```python
from build123d import *

# Parameters (mm, degrees)
SKETCH5_R           = 11.5
BOSS_EXTRUDE2_DEPTH = 3
BOSS_EXTRUDE1_DEPTH = 3
SKETCH3_W           = 6
SKETCH3_H           = 3
SKETCH3_W_2         = 3
SKETCH3_H_2         = 6
CUT_EXTRUDE1_DEPTH  = 3
SKETCH6_R           = 1.35
CUT_EXTRUDE3_DEPTH  = 3


with BuildPart() as part:
    # Sketch5 → Boss-Extrude2 (new body)
    with BuildSketch(Plane(origin=(0, 0, 0), x_dir=(1, 0, 0), z_dir=(0, 1, 0))):
        with Locations(Location((0, 0, 0), (0, 0, 270))):
            Circle(SKETCH5_R)
    extrude(amount=BOSS_EXTRUDE2_DEPTH)

    # Sketch1 → Boss-Extrude1 (add)
    with BuildSketch(Plane(origin=(0, 0, 0), x_dir=(1, 0, 0), z_dir=(0, 1, 0))):
        Polygon((0, 16), (-1.75, 11), (1.75, 11), align=None)
        Polygon((5.195191507, 15.133075867), (1.916513988, 10.97221373), (5.226874334, 9.835765588), align=None)
        Polygon((9.827403403, 12.62624815), (5.375343948, 9.755417851), (8.137335731, 7.605673356), align=None)
        Polygon((13.394663652, 8.75117053), (8.251671984, 7.481471076), (10.165990538, 4.551388402), align=None)
        Polygon((15.510404255, 3.927767794), (10.233803323, 4.396790824), (11.093002528, 1.003889893), align=None)
        Polygon((15.945351888, -1.321269528), (11.106943278, 0.835650063), (10.817915568, -2.652395663), align=None)
        Polygon((14.652373226, -6.427126794), (10.776473586, -2.81604635), (9.3705396, -6.021252993), align=None)
        Polygon((11.771582571, -10.836505146), (9.278205768, -6.162580444), (6.907720267, -8.737614132), align=None)
        Polygon((7.615158289, -14.071580019), (6.774500388, -8.841303325), (3.696342259, -10.507119201), align=None)
        Polygon((2.633513444, -15.781780854), (3.536672774, -10.561933804), (0.084408212, -11.13801487), align=None)
        Polygon((-2.633513444, -15.781780854), (-0.084408212, -11.13801487), (-3.536672774, -10.561933804), align=None)
        Polygon((-7.615158289, -14.071580019), (-3.696342259, -10.507119201), (-6.774500388, -8.841303325), align=None)
        Polygon((-11.771582571, -10.836505146), (-6.907720267, -8.737614132), (-9.278205768, -6.162580444), align=None)
        Polygon((-14.652373226, -6.427126794), (-9.3705396, -6.021252993), (-10.776473586, -2.81604635), align=None)
        Polygon((-15.945351888, -1.321269528), (-10.817915568, -2.652395663), (-11.106943278, 0.835650063), align=None)
        Polygon((-15.510404255, 3.927767794), (-11.093002528, 1.003889893), (-10.233803323, 4.396790824), align=None)
        Polygon((-13.394663652, 8.75117053), (-10.165990538, 4.551388402), (-8.251671984, 7.481471076), align=None)
        Polygon((-9.827403403, 12.62624815), (-8.137335731, 7.605673356), (-5.375343948, 9.755417851), align=None)
        Polygon((-5.195191507, 15.133075867), (-5.226874334, 9.835765588), (-1.916513988, 10.97221373), align=None)
    extrude(amount=BOSS_EXTRUDE1_DEPTH)

    # Sketch3 → Cut-Extrude1 (cut)
    with BuildSketch(Plane(origin=(0, 0, 0), x_dir=(1, 0, 0), z_dir=(0, 1, 0))):
        with Locations((0, 7.5)):
            Rectangle(SKETCH3_W, SKETCH3_H)
        with Locations((7.5, 0)):
            Rectangle(SKETCH3_W_2, SKETCH3_H_2)
        with Locations((0, -7.5)):
            Rectangle(SKETCH3_W, SKETCH3_H)
        with Locations((-7.5, 0)):
            Rectangle(SKETCH3_W_2, SKETCH3_H_2)
    extrude(amount=CUT_EXTRUDE1_DEPTH, mode=Mode.SUBTRACT)

    # Sketch6 → Cut-Extrude3 (cut)
    with BuildSketch(Plane(origin=(0, 3, 0), x_dir=(1, 0, 0), z_dir=(0, 1, 0))):
        with Locations(Location((0, 0, 0), (0, 0, 270))):
            Circle(SKETCH6_R)
    extrude(amount=-CUT_EXTRUDE3_DEPTH, mode=Mode.SUBTRACT)


solid = part.part
```
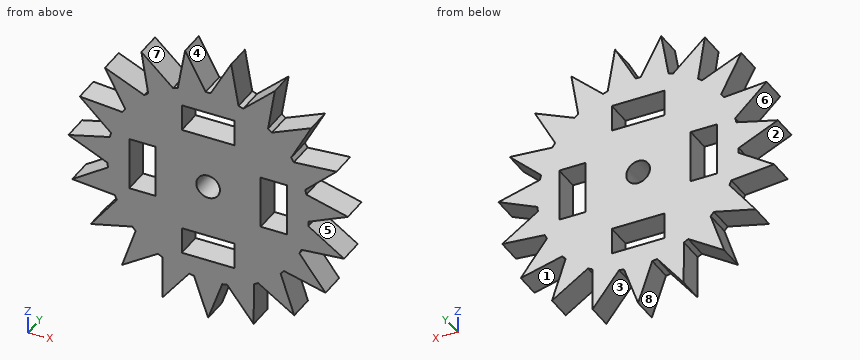
Could you check a few things on this model? Use its own coordinates, in mm. Face numbers are marked on the shaded views. A direction names the side the tool comes from. Round coordinates to 2 decimals unless told otherwise and drop trailing zeros. Write each loop counter-clockwise with the first axis right and the second up, starting at its lowest first coordinate (ties: lowest second). Pieces come first, ordered by that corner, then holes. Notation, with made-up numbers: M -4,60 L 35,60 A12 cw 35,75 Z; hole C 64,29.5 d5. An arc over 180 degrees is marked long. Write each question's results on one line, items separated by ' | '. Start each with the question number.
1. Imagine slicing it at A-A on z = 2. List the corners of the cut face in (x, y) for me, and give its area (3 significant figures).
2. On a 3-axis mill with a long thin cutter (end or side, diameter ignored), from which of +Z, -Z, +X, -X, +Y, -Y can I reach the whole of each face in a straight line? I mean the marked faces 1, 2, 3, 4 and 5. Say none if no direction works.
3. Imagine slicing it at C-C on y = 1.2. Count the separate pieces of the cut face and the enclosed holes in it, and give its area (3 significant figures).
4. I need wall thicknesses on L1, parallel to X at y = 0.85, z = 12; L2, parallel to X at y = 1.45, z = 0; L3, parallel to Z at x = -10.5, y = 2.3. Which ranges of each line are inside material? Lowest first, please. Write a range as from..to.
5. Imagine slicing it at B-B on x = -12.5. List the corners of the cut face in (y, z) for me.
6. I'm going to push flat-ended pins straight in: pin 1 Ø0.9 at (y, z) = (1.5, -0.5) entering from +X; pin 2 Ø0.9 at (y, z) = (1, 0.5) entering from -X; pin 3 Ø1.5 at (x, y) = (-8, 2) entering from -Z. Where does each tip first touch, or does it pass through?
7. Thinking about a two-plate mould opening in Z: for the marked faces 6, 7 and 8, which applies, +Z half, -Z half, draft (parallel to the pull), parting line (faces both ways), or undercut?
Result sheet:
1) outline: M -13.33,0 L -9,0 L -9,3 L -13.33,3 Z; M -6,0 L 6,0 L 6,3 L -6,3 Z; M 9,0 L 13.33,0 L 13.33,3 L 9,3 Z | area: 62.0 mm^2
2) face 1: +Y, -Y | face 2: -X, +Y, -Y | face 3: -Z, +Y, -Y | face 4: +Z, +Y, -Y | face 5: +X, +Y, -Y
3) separate pieces: 1 | enclosed holes: 5 | area: 475 mm^2
4) L1: x = -7.28..-5.34, -3.29..-0.56, 0.56..3.29, 5.34..7.28 | L2: x = -12.98..-9, -6..-1.35, 1.35..6, 9..12.98 | L3: z = -8.04..-4.99, -4.69..6.11, 8.45..10.29
5) outline: M 0,-8.53 L 3,-8.53 L 3,-7.59 L 0,-7.59 Z; M 0,-4.2 L 3,-4.2 L 3,-1.94 L 0,-1.94 Z; M 0,-0.21 L 3,-0.21 L 3,2.22 L 0,2.22 Z; M 0,4.42 L 3,4.42 L 3,6.26 L 0,6.26 Z
6) pin 1: stops at x = 12.87 | pin 2: stops at x = -15.11 | pin 3: stops at z = -11.93
7) face 6: undercut | face 7: +Z half | face 8: -Z half
